Part model, mm, in its own coordinate system. A direction names the side the tool comes from. Give positions to 0.01 mm unless a question says otherwise; leave off trailing zeros. Loops run counter-clockwise (first coordinate to the right, second up) from the corner with the lowest first, then second, coordinate; pieces in that order, holes last. Notation, with made-up numbers: (82.5, 74) -> (107.5, 74) arc R17 ccw to (107.5, 95) -> close; hole circle Ø4 at (6.25, 33.25). An arc over 180 degrees is marked (long way). Write item = value, one per line.
from build123d import *

# Parameters (mm, degrees)
MIDDLE_SKETCH_W               = 5.5
MIDDLE_SKETCH_H               = 16
MIDDLE_SKETCH_W_2             = 26
MIDDLE_SKETCH_H_2             = 9
MIDDLE_EXTRUDE_DEPTH          = 1.5
OFFSHOOT_RIGHT_PLANE_SKETCH_W = 16
OFFSHOOT_RIGHT_PLANE_SKETCH_H = 21.33030278
RIGHT_OFFSHOOT_EXTRUDE_DEPTH  = 1.5
OFFSHOOT_LEFT_PLANE_SKETCH_W  = 16
OFFSHOOT_LEFT_PLANE_SKETCH_H  = 21.33030278
LEFT_OFFSHOOT_EXTRUDE_DEPTH   = 1.5
F_2_7_2_7_DIAMETER_HOLE1_D    = 2.7
F_2_7_2_7_DIAMETER_HOLE2_D    = 2.7
F_1_8_1_8_DIAMETER_HOLE1_D    = 1.8


with BuildPart() as part:
    # Middle Sketch → Middle Extrude (new body)
    with BuildSketch(Plane(origin=(0, 0, 0), x_dir=(1, 0, 0), z_dir=(0, 1, 0))):
        with Locations((-22.75, -3.5)):
            Rectangle(MIDDLE_SKETCH_W, MIDDLE_SKETCH_H)
        Polygon((-20, -11.5), (-20, 4.5), (-13, 4.5), (-13, -4.5), align=None)
        Rectangle(MIDDLE_SKETCH_W_2, MIDDLE_SKETCH_H_2)
        Polygon((13, 4.5), (20, 4.5), (20, -11.5), (13, -4.5), align=None)
        with Locations((22.75, -3.5)):
            Rectangle(MIDDLE_SKETCH_W, MIDDLE_SKETCH_H)
    extrude(amount=MIDDLE_EXTRUDE_DEPTH)

    # Offshoot Right Plane Sketch → Right Offshoot Extrude (add)
    with BuildSketch(Plane(origin=(12.75, -12.75, 0), x_dir=(0, 0, -1), z_dir=(0.707106781, -0.707106781, 0))):
        with BuildLine():
            Line((4.5, 39.3615257), (-11.5, 39.3615257))
            ThreePointArc((-11.5, 39.3615257), (-3.5, 41.03122292), (4.5, 39.3615257))
        make_face()
        with Locations((-3.5, 28.69637431)):
            Rectangle(OFFSHOOT_RIGHT_PLANE_SKETCH_W, OFFSHOOT_RIGHT_PLANE_SKETCH_H)
    extrude(amount=-RIGHT_OFFSHOOT_EXTRUDE_DEPTH)

    # Offshoot Left Plane Sketch → Left Offshoot Extrude (add)
    with BuildSketch(Plane(origin=(-12.75, -12.75, 0), x_dir=(0, 0, -1), z_dir=(-0.707106781, -0.707106781, 0))):
        with Locations((-3.5, -28.69637431)):
            Rectangle(OFFSHOOT_LEFT_PLANE_SKETCH_W, OFFSHOOT_LEFT_PLANE_SKETCH_H)
        with BuildLine():
            ThreePointArc((4.5, -39.3615257), (-3.5, -41.03122292), (-11.5, -39.3615257))
            Line((-11.5, -39.3615257), (4.5, -39.3615257))
        make_face()
    extrude(amount=-LEFT_OFFSHOOT_EXTRUDE_DEPTH)

    # Ø2.7 (2.7) Diameter Hole1 (through all)
    with Locations(Plane(origin=(-11.689339828, -11.689339828, 0), x_dir=(0.707106781, -0.707106781, 0), z_dir=(0.707106781, 0.707106781, 0))):
        with Locations((-37.03122292, -8.5), (-25.03122292, 1.5)):
            Hole(F_2_7_2_7_DIAMETER_HOLE1_D / 2)

    # Ø2.7 (2.7) Diameter Hole2 (through all)
    with Locations(Plane(origin=(11.689339828, -11.689339828, 0), x_dir=(0.707106781, 0.707106781, 0), z_dir=(-0.707106781, 0.707106781, 0))):
        with Locations((25.03122292, 1.5), (37.03122292, -8.5)):
            Hole(F_2_7_2_7_DIAMETER_HOLE2_D / 2)

    # Ø1.8 (1.8) Diameter Hole1 (through all)
    with Locations(Plane(origin=(0, 1.5, 0), x_dir=(1, 0, 0), z_dir=(0, 1, 0))):
        with Locations((-10.5, 0), (10.5, 0)):
            Hole(F_1_8_1_8_DIAMETER_HOLE1_D / 2)


solid = part.part
1) Pull direction Z, two halves, no side cores. Call faces 4 (the face through (-30, 6, 11.5)), 5 (the face through (9.64, 0.74, -0.27)), 6 (the face through (0, 1.5, 2)): pulls with the +Z half, pulls with the -Z half, needs draft (parallel to the pull), parting line crosses it, or undercut.
Resolved:
face_4 = pulls with the +Z half
face_5 = undercut
face_6 = needs draft
2) Which spindle directions (+Z, -Z, +X, -X, +Y, -Y) get a long thin tool onto all of the face, cutting with end or side? Do faces 1 (the face through (16.5, 0.7, 8)), 2 (the face through (-33.5, 8, 3.6)), 3 (the face through (-32.68, 9.3, 3.61)). Say none if no direction does.
Resolved:
face_1 = +Z, +Y, -Y
face_2 = +Z, -Z, -X, -Y
face_3 = +Z, -Z, +Y
3) Slice it at A-A, the plane x = -10.5. List the corners of the cut face in (y, z).
Resolved:
outline = (0, -4.5) -> (1.5, -4.5) -> (1.5, -0.9) -> (0, -0.9) -> close; (0, 0.9) -> (1.5, 0.9) -> (1.5, 4.5) -> (0, 4.5) -> close
4) Slice it at B-B, the plane z = 5.5. List the corners of the cut face in (x, y).
Resolved:
outline = (-41.69, 16.19) -> (-25.5, 0) -> (-14, 0) -> (-14, 1.5) -> (-24.88, 1.5) -> (-40.63, 17.25) -> close; (14, 0) -> (25.5, 0) -> (41.69, 16.19) -> (40.63, 17.25) -> (24.88, 1.5) -> (14, 1.5) -> close
5) Drill centre lines: line 1 along Z through (x, y) = (-10.5, 0.9); line 2 along Y through (x, z) = (11.5, 1.25); line 3 along X through (y, z) = (1.25, 9). Where is each one in solid material? Low to high. Write a range as [from, to].
Resolved:
line_1 = [-4.5, -0.9], [0.9, 4.5]
line_2 = [0, 1.5]
line_3 = [-26.75, -17.5], [17.5, 26.75]
6) Slice it at C-C, the plane y = 10. List the corners of the cut face in (x, z), and give its area (3 significant figures).
Resolved:
outline = (-35.5, -4.5) -> (-33.38, -4.5) -> (-33.38, 11.5) -> (-35.5, 11.5) -> close; (33.38, -4.5) -> (35.5, -4.5) -> (35.5, 11.5) -> (33.38, 11.5) -> close
area = 67.9 mm²
7) Drop flat-ended pins along their axis: P1, Ø6, axis at y = 9, z = 6, coming from the +X side; P2, Ø8, axis at x = -9.5, z = 1, coming from the +Y side; P3, Ø2, axis at y = 2.5, z = 5, coming from the +X side; P4, Ø1.4, axis at x = -10.5, z = 0, coming from the -Y side. Give the stop position or say it passes through.
Resolved:
P1 = 37.5
P2 = 1.5
P3 = 29
P4 = through
